from build123d import *

# Parameters (mm, degrees)
SKETCH1_W           = 100
SKETCH1_H           = 100
BOSS_EXTRUDE1_DEPTH = 180
SKETCH2_R           = 34.257790197
BOSS_EXTRUDE2_DEPTH = 350
SKETCH3_W           = 152.006357392
SKETCH3_H           = 282.452416457
CUT_EXTRUDE2_DEPTH  = 400
CUT_EXTRUDE3_DEPTH  = 400
CUT_EXTRUDE4_DEPTH  = 400
CUT_EXTRUDE5_DEPTH  = 400
SKETCH7_W           = 160.159381639
SKETCH7_H           = 147.362276113
CUT_EXTRUDE6_DEPTH  = 400
SKETCH8_W           = 147.310744502
SKETCH8_H           = 162.038906966
CUT_EXTRUDE7_DEPTH  = 400
SKETCH9_R           = 31.847293423
CUT_EXTRUDE8_DEPTH  = 400
SKETCH10_W          = 140.220962397
SKETCH10_H          = 212.033531124
CUT_EXTRUDE9_DEPTH  = 400
SKETCH11_R          = 13.603137886
CUT_EXTRUDE11_DEPTH = 15
SKETCH12_R          = 12.495422516
BOSS_EXTRUDE3_DEPTH = 15
SKETCH13_R          = 1.594865099
BOSS_EXTRUDE4_DEPTH = 4
SKETCH14_W          = 100.74862993
SKETCH14_H          = 110.555003588
CUT_EXTRUDE13_DEPTH = 400
BOSS_EXTRUDE5_DEPTH = 1
SKETCH16_W          = 42.108585165
SKETCH16_H          = 30.458347221
BOSS_EXTRUDE6_DEPTH = 5
SKETCH17_W          = 18.669530869
SKETCH17_H          = 22.4027039
BOSS_EXTRUDE7_DEPTH = 1
SKETCH18_W          = 4.907623399
SKETCH18_H          = 5.170746831
SKETCH18_W_2        = 3.981473695
SKETCH18_H_2        = 5.451349552
BOSS_EXTRUDE8_DEPTH = 1
CUT_EXTRUDE14_DEPTH = 2


with BuildPart() as part:
    # Sketch1 → Boss-Extrude1 (new body)
    with BuildSketch(Plane(origin=(0, 0, 0), x_dir=(1, 0, 0), z_dir=(0, 1, 0))):
        with Locations((-50, 50)):
            Rectangle(SKETCH1_W, SKETCH1_H)
    extrude(amount=BOSS_EXTRUDE1_DEPTH)

    # Sketch2 → Boss-Extrude2 (add, symmetric)
    with BuildSketch(Plane(origin=(0, 180, 0), x_dir=(1, 0, 0), z_dir=(0, 1, 0))):
        with Locations(Location((-51.377291833, 49.076536384, 0), (0, 0, 270))):
            Circle(SKETCH2_R)
    extrude(amount=BOSS_EXTRUDE2_DEPTH, both=True)

    # Sketch3 → Cut-Extrude2 (cut)
    with BuildSketch(Plane(origin=(0, 0, 0), x_dir=(0, 0, -1), z_dir=(1, 0, 0))):
        with Locations((57.419900112, 502.274302507)):
            Rectangle(SKETCH3_W, SKETCH3_H)
    extrude(amount=-CUT_EXTRUDE2_DEPTH, mode=Mode.SUBTRACT)

    # Sketch4 → Cut-Extrude3 (cut)
    with BuildSketch(Plane(origin=(0, 0, 0), x_dir=(0, 0, -1), z_dir=(1, 0, 0))):
        Polygon((12.981970869, 0), (-8.994244796, 25.828096003), (-18.564506014, -15.259465835), align=None)
        Polygon((85.072517936, -1.448103984), (109.237639161, 19.113145112), (115.920034239, -3.267382694), align=None)
        Polygon((12.981970869, 180), (-8.994244796, 148.537596011), (-15.418178585, 193.219274892), align=None)
        Polygon((85.072517936, 181.854312784), (103.841225373, 159.795920888), (106.132549481, 198.647393934), align=None)
    extrude(amount=-CUT_EXTRUDE3_DEPTH, mode=Mode.SUBTRACT)

    # Sketch5 → Cut-Extrude4 (cut)
    with BuildSketch(Plane.XY):
        Polygon((-85.623287335, 0), (-106.370377984, 21.426392531), (-122.288861874, 3.209259887), (-93.526345261, -19.884701759), align=None)
        Polygon((-15.694988751, 0), (0, 15.257385304), (12.122677088, 15.257385304), (10.563067769, -19.884701759), align=None)
        Polygon((-87.166490339, 180.248071029), (-106.370377984, 151.29108453), (-117.705469457, 200.501115102), align=None)
        Polygon((-15.694988751, 180.248071029), (7.833767065, 153.279557508), (0, 193.941208308), align=None)
    extrude(amount=-CUT_EXTRUDE4_DEPTH, mode=Mode.SUBTRACT)

    # Sketch6 → Cut-Extrude5 (cut)
    with BuildSketch(Plane(origin=(0, 180, 0), x_dir=(1, 0, 0), z_dir=(0, 1, 0))):
        Polygon((-112.386997555, 28.400400964), (-64.261264503, -10.212759359), (-84.406366528, -15.51192827), (-124.649689542, -15.51192827), align=None)
        Polygon((-97.065537028, 135.861756084), (-119.37552445, 77.792688888), (-118.043343626, 64.347606737), (-66.428694172, 110.575168787), align=None)
        Polygon((-24.69640689, -21.815840769), (11.092108798, -8.97361337), (17.428316417, 32.393768119), (-38.531576846, -11.139157378), align=None)
        Polygon((-17.445484601, 140.804394854), (35.417473102, 107.262520599), (9.305452855, 72.996438725), (-31.724385352, 103.625272537), align=None)
    extrude(amount=-CUT_EXTRUDE5_DEPTH, mode=Mode.SUBTRACT)

    # Sketch7 → Cut-Extrude6 (cut)
    with BuildSketch(Plane.XY):
        with Locations((-66.123258915, -136.36252694)):
            Rectangle(SKETCH7_W, SKETCH7_H)
    extrude(amount=-CUT_EXTRUDE6_DEPTH, mode=Mode.SUBTRACT)

    # Sketch8 → Cut-Extrude7 (cut)
    with BuildSketch(Plane.XY):
        with Locations((-53.541153336, 332.448287589)):
            Rectangle(SKETCH8_W, SKETCH8_H)
    extrude(amount=-CUT_EXTRUDE7_DEPTH, mode=Mode.SUBTRACT)

    # Sketch9 → Cut-Extrude8 (cut)
    with BuildSketch(Plane(origin=(0, 251.428834106, 0), x_dir=(1, 0, 0), z_dir=(0, 1, 0))):
        with Locations(Location((-50.808993157, 49.032036374, 0), (0, 0, 270))):
            Circle(SKETCH9_R)
    extrude(amount=-CUT_EXTRUDE8_DEPTH, mode=Mode.SUBTRACT)

    # Sketch10 → Cut-Extrude9 (cut)
    with BuildSketch(Plane.ZY.offset(100)):
        with Locations((14.299084536, 180.100625535)):
            Rectangle(SKETCH10_W, SKETCH10_H)
    extrude(amount=-CUT_EXTRUDE9_DEPTH, mode=Mode.SUBTRACT)

    # Sketch11 → Cut-Extrude11 (cut)
    with BuildSketch(Plane.ZY.offset(100)):
        with Locations((-50.413251954, 76.264646142)):
            Circle(SKETCH11_R)
    extrude(amount=-CUT_EXTRUDE11_DEPTH, mode=Mode.SUBTRACT)

    # Sketch12 → Boss-Extrude3 (add)
    with BuildSketch(Plane.ZY.offset(85)):
        with Locations(Location((-50.658800768, 76.222522328, 0), (0, 0, 114.353089558))):
            Circle(SKETCH12_R)
    extrude(amount=BOSS_EXTRUDE3_DEPTH)

    # Sketch13 → Boss-Extrude4 (add)
    with BuildSketch(Plane(origin=(-85, 0, 0), x_dir=(0, 0, -1), z_dir=(1, 0, 0))):
        with Locations(Location((49.945205578, 75.944780088, 0), (0, 0, 180))):
            Circle(SKETCH13_R)
    extrude(amount=BOSS_EXTRUDE4_DEPTH)

    # Sketch14 → Cut-Extrude13 (cut)
    with BuildSketch(Plane.ZY.offset(100)):
        with Locations((-65.350029467, 250.603414818)):
            Rectangle(SKETCH14_W, SKETCH14_H)
    extrude(amount=-CUT_EXTRUDE13_DEPTH, mode=Mode.SUBTRACT)

    # Sketch15 → Boss-Extrude5 (add)
    with BuildSketch(Plane.ZY.offset(100)):
        Polygon((-18.461827727, 14.847435435), (-80.507743362, 14.847435435), (-80.507743362, 160.896793159), (-55.811396663, 160.896793159), (-55.811396663, 74.083859973), (-18.461827727, 74.083859973), align=None)
    extrude(amount=BOSS_EXTRUDE5_DEPTH)

    # Sketch16 → Boss-Extrude6 (add)
    with BuildSketch(Plane.ZY.offset(101)):
        with Locations((-48.07732297, 45.136437142)):
            Rectangle(SKETCH16_W, SKETCH16_H)
    extrude(amount=BOSS_EXTRUDE6_DEPTH)

    # Sketch17 → Boss-Extrude7 (add)
    with BuildSketch(Plane.ZY.offset(101)):
        with Locations((-67.04663872, 130.409241603)):
            Rectangle(SKETCH17_W, SKETCH17_H)
    extrude(amount=BOSS_EXTRUDE7_DEPTH)

    # Sketch18 → Boss-Extrude8 (add)
    with BuildSketch(Plane.ZY.offset(102)):
        with Locations((-71.625108618, 130.213401885)):
            Rectangle(SKETCH18_W, SKETCH18_H)
        with Locations((-62.297675883, 129.867186512)):
            Rectangle(SKETCH18_W_2, SKETCH18_H_2)
    extrude(amount=BOSS_EXTRUDE8_DEPTH)

    # Sketch19 → Cut-Extrude14 (cut)
    with BuildSketch(Plane.ZY.offset(102)):
        Polygon((-66.976455081, 134.868836652), (-73.7929295, 134.868836652), (-73.7929295, 134.108269479), (-74.571872104, 134.108269479), (-74.571872104, 140.512729543), (-73.7929295, 140.512729543), (-72.165965418, 140.512729543), (-72.233411796, 137.421948277), (-71.48458153, 137.421948277), (-71.410861795, 140.512729543), (-69.158339735, 140.504865112), (-69.158339735, 137.421948277), (-68.22174926, 137.421948277), (-68.22174926, 140.567922793), (-65.426885805, 140.567922793), (-65.515241968, 137.446210948), (-64.714122339, 137.446210948), (-64.714122339, 140.567922793), (-62.410871788, 140.567922793), (-62.410871788, 137.210126003), (-61.403493639, 137.210126003), (-61.403493639, 140.631129361), (-58.889974549, 140.631129361), (-58.889974549, 136.595539338), (-59.698319644, 136.595539338), (-59.698319644, 139.99489006), (-60.695848378, 139.984078324), (-60.695848378, 136.667717235), (-63.090112056, 136.667717235), (-63.090112056, 139.979723883), (-64.00479018, 139.979723883), (-64.00479018, 136.667717235), (-66.334605538, 136.667717235), (-66.334605538, 139.902697072), (-67.48995239, 139.902697072), (-67.48995239, 136.667717235), (-70.008746759, 136.667717235), (-70.008746759, 139.902697072), (-70.709698815, 139.902697072), (-70.783897489, 136.693128041), (-72.921241048, 136.693128041), (-72.921241048, 139.545601992), (-73.7929295, 139.545601992), (-73.7929295, 135.423339258), (-66.976455081, 135.49721976), align=None)
    extrude(amount=-CUT_EXTRUDE14_DEPTH, mode=Mode.SUBTRACT)


solid = part.part
For this review, take the finished solid that the model builds, in its own axes (mm). A direction names the side the tool comes from. Coordinates: 2 decimals unless noted, no trailing zeros. Write each loop counter-clockwise with the first axis right and the second up, starting at its lowest first coordinate (ties: lowest second). Pieces come first, ordered by that corner, then holes. Notation, with made-up numbers: (72, -22.75) -> (119, -22.75) arc R20 cw to (119, -16.75) -> close; hole circle Ø9 at (85.5, 42.25). An arc over 180 degrees is marked (long way). Write each question's results on one line, items separated by ' | '. Start each with the question number.
1) For faces 5 (the face through (-25, 0, -72)), 6 (the face through (-103, 45, -27.023)), 7 (the face through (-13.246, 90.863, -89.831)), list the 3-axis set-ups (+Z, -Z, +X, -X, +Y, -Y) from which the entire face can be reached by the end or side of a thin tool; tool diameter is ignored.
2) Insertion check: pin 1 (0.5 mm diameter, centred on x = -102.5, z = -62, fed in from +Y); pin 2 (6 mm diameter, centred on y = -34.5, z = -62, fed in from -X); pin 3 (0.8 mm diameter, centred on x = -102.5, y = 130.5, fed in from +Z); pin 4 (6 mm diameter, centred on x = -24, z = -47.5, fed in from -Y). Each pin has a flat end and moves straight along its axis. Give the tip position at first contact, or say it passes through.
3) Consider section C-C (y = 45). Write out the cut boundary in (x, z), plus the area to 3 significant figures.
4) Consider section D-D (z = -34). Write out the cut boundary in (x, y).
5) Consider section B-B (z = -23.5). Write out the cut boundary in (x, y).
6) The part is to be moulded in two halves that separate along Z. For faces 1 (the face through (-49.9, 7.5, -6.6)), 2 (the face through (-92.395, 64.623, -46.012)), 3 (the face through (-100, 64, -54)), 4 (the face through (-52, 180, -85)), say which applies: +Z half, -Z half, draft (parallel to the pull), parting line (faces both ways), or undercut.
7) Wall thickness on L1, parallel to X at y = 61, z = -20.5; L2, parallel to Y at x = -22.5, z = -27; L3, parallel to X at y = 93.5, z = -64: over which ranges is each line inside the solid? List them lowest first. Write a range as [from, to].
8) Consider section A-A (x = -32.5). Write out the cut boundary in (y, z).
Geometry says:
1) face 5: -Y | face 6: +Z, -X, +Y, -Y | face 7: -Z, +X, +Y, -Y
2) pin 1: y = 132.59 | pin 2: x = -84.17 | pin 3: z = -60.31 | pin 4: through
3) outline: (-106, -69.13) -> (-101, -69.13) -> (-101, -80.51) -> (-100, -80.51) -> (-78.24, -100) -> (-26.87, -100) -> (0, -79.94) -> (0, -18.84) -> (-24.21, 0) -> (-76.99, 0) -> (-100, -18.46) -> (-101, -18.46) -> (-101, -27.02) -> (-106, -27.02) -> close; hole circle Ø63.69 at (-50.81, -49.03) | area: 6,160 mm^2
4) outline: (-106, 29.91) -> (-101, 29.91) -> (-101, 14.85) -> (-100, 14.85) -> (-85.62, 0) -> (-82.14, 0) -> (-82.14, -62.68) -> (-78.89, -62.68) -> (-78.89, 74.08) -> (-101, 74.08) -> (-101, 60.37) -> (-106, 60.37) -> close; (-22.73, -62.68) -> (-20.62, -62.68) -> (-20.62, 0) -> (-15.69, 0) -> (0, 15.26) -> (0, 74.08) -> (-22.73, 74.08) -> close
5) outline: (-101, 14.85) -> (-100, 14.85) -> (-85.62, 0) -> (-74.17, 0) -> (-74.17, -62.68) -> (-69.84, -62.68) -> (-69.84, 74.08) -> (-101, 74.08) -> close; (-31.77, -62.68) -> (-28.59, -62.68) -> (-28.59, 0) -> (-15.69, 0) -> (0, 15.26) -> (0, 74.08) -> (-31.77, 74.08) -> close
6) face 1: +Z half | face 2: undercut | face 3: undercut | face 4: draft
7) L1: [-101, -64.96], [-36.66, 0] | L2: [0, 74.08] | L3: [-101, -78.92], [-22.7, 0]
8) outline: (-62.68, -77.66) -> (0, -77.66) -> (0, -86.77) -> (11.25, -100) -> (164.31, -100) -> (180, -86.65) -> (180, -77.66) -> (195.33, -77.66) -> (195.33, -75.09) -> (-62.68, -75.09) -> close; (-62.68, -22.97) -> (74.08, -22.97) -> (74.08, 0) -> (15.26, 0) -> (0, -12.98) -> (0, -20.49) -> (-62.68, -20.49) -> close
